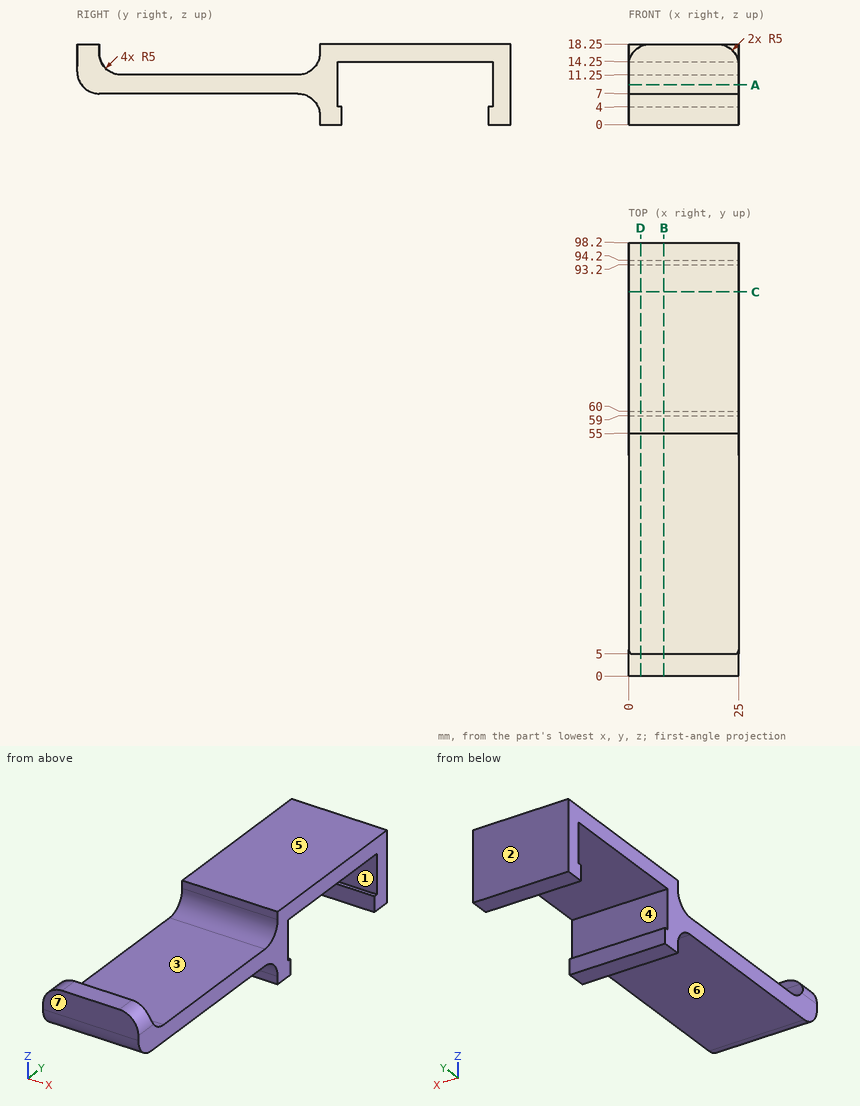
For this review, use the dimensioned drawing (mm, ordinates from the lowest corner) and the shaded views. A direction names the side the tool comes from. Coordinates: 2 decimals unless noted, no trailing zeros. Order: outer loops, then holes, each group sorted by start corner. A loop starts at its lowest first (then second) coordinate and runs counter-clockwise, first axis right, second up. Notation, with made-up numbers: (11, 0.25) - (67, 0.25) arc R12 cw to (67, 4.25) - close; hole circle Ø5 at (-35, 67). An arc over 180 degrees is marked (long way). Answer as a JSON object with one key per item and string values. Group by question number.
1. For the marked faces 1, 2 and 3, list the 3-axis set-ups (+Z, -Z, +X, -X, +Y, -Y) from which the entire face can be reached by the end or side of a thin tool; tool diameter is ignored.
2. Clearance check with flat-ended pins moving along their axes: P1, Ø10, axis at y = 12.5, z = 4.5, coming from the -X side; P2, Ø3, axis at x = 7, z = 3, coming from the -Y side; P3, Ø6, axis at y = 37, z = 2.5, coming from the -X side; P4, Ø2, axis at x = 7.5, z = 1, coming from the -Y side. State where each tip first meets the part, or that it passes through.
3. For probe 1 along Y at (x, z) = (10.5, 16.5); probe 2 along Y at (x, z) = (4.5, 9); probe 3 along Z at (x, y) = (11.25, 12), list the stretches that pass through material, from the lowest coordinate up.
4. We need section D-D on x = 2.75. State the section outline as (y, z) points, then the cut area to 3 significant figures.
5. The part is to be moulded in two halves that separate along Z. For the marked faces 4, 5, 6 and 7, say which applies: pulls with the +Z half, pulls with the -Z half, needs draft (parallel to the pull), parting line crosses it, or undercut.
6. We need section C-C on y = 87. State the section outline as (x, z) points, then the cut area to 3 significant figures.
7. We need section A-A on z = 9. State the section outline as (x, y) points, then the cut area to 3 significant figures.
8. We need section B-B on x = 8. State the section outline as (y, z) points, then the cut area to 3 significant figures.
Final values:
{
 "1": {"face 1": "+X, -X", "face 2": "+Z, -Z, +X, -X, +Y", "face 3": "+Z, +X, -X"},
 "2": {"P1": "x = 0", "P2": "y = 54.33", "P3": "through", "P4": "y = 55"},
 "3": {"probe 1": "0 to 5, 55 to 98.2", "probe 2": "1 to 59, 94.2 to 98.2", "probe 3": "7 to 11.25"},
 "4": {"outline": "(0, 12) arc R5 ccw to (5, 7) - (50, 7) arc R5 cw to (55, 2) - (55, 0) - (60, 0) - (60, 4) - (59, 4) - (59, 14.25) - (94.2, 14.25) - (94.2, 4) - (93.2, 4) - (93.2, 0) - (98.2, 0) - (98.2, 18.25) - (55, 18.25) - (55, 16.25) arc R5 cw to (50, 11.25) - (10, 11.25) arc R5 cw to (5, 16.25) - (5, 17.72) - (0, 17.72) - close", "area": "572 mm²"},
 "5": {"face 4": "undercut", "face 5": "pulls with the +Z half", "face 6": "pulls with the -Z half", "face 7": "needs draft"},
 "6": {"outline": "(0, 14.25) - (25, 14.25) - (25, 18.25) - (0, 18.25) - close", "area": "100 mm²"},
 "7": {"outline": "(0, 1) - (25, 1) - (25, 59) - (0, 59) - close; (0, 94.2) - (25, 94.2) - (25, 98.2) - (0, 98.2) - close", "area": "1,550 mm²"},
 "8": {"outline": "(0, 12) arc R5 ccw to (5, 7) - (50, 7) arc R5 cw to (55, 2) - (55, 0) - (60, 0) - (60, 4) - (59, 4) - (59, 14.25) - (94.2, 14.25) - (94.2, 4) - (93.2, 4) - (93.2, 0) - (98.2, 0) - (98.2, 18.25) - (55, 18.25) - (55, 16.25) arc R5 cw to (50, 11.25) - (10, 11.25) arc R5 cw to (5, 16.25) - (5, 18.25) - (0, 18.25) - close", "area": "574 mm²"}
}
